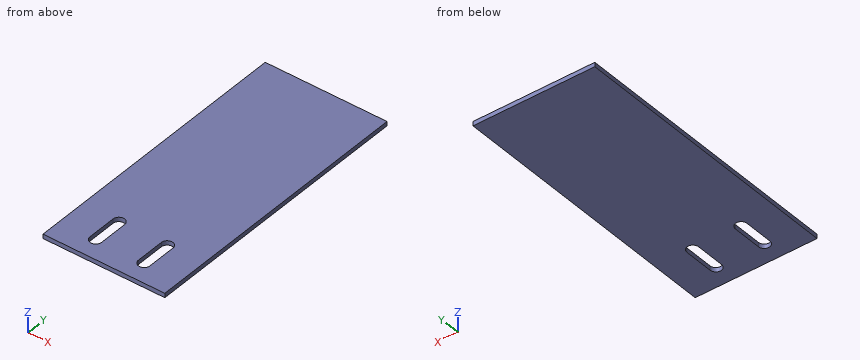
from build123d import *

# Parameters (mm, degrees)
SKETCH1_W           = 126
SKETCH1_H           = 290
BOSS_EXTRUDE2_DEPTH = 4.5


with BuildPart() as part:
    # Sketch1 → Boss-Extrude2 (new body)
    with BuildSketch(Plane.XY):
        Rectangle(SKETCH1_W, SKETCH1_H)
        with BuildLine():
            Line((-19, -109), (-19, -124))
            ThreePointArc((-19, -124), (-25, -130), (-31, -124))
            Line((-31, -124), (-31, -94))
            ThreePointArc((-31, -94), (-25, -88), (-19, -94))
            Line((-19, -94), (-19, -109))
        make_face(mode=Mode.SUBTRACT)
        with BuildLine():
            ThreePointArc((31, -124), (25, -130), (19, -124))
            Line((19, -124), (19, -94))
            ThreePointArc((19, -94), (25, -88), (31, -94))
            Line((31, -94), (31, -124))
        make_face(mode=Mode.SUBTRACT)
    extrude(amount=BOSS_EXTRUDE2_DEPTH)


solid = part.part
Input: part model. Units: mm. Frame: model coordinates. Coordinates: 2 decimals unless noted, no trailing zeros. Loops run counter-clockwise (first coordinate to the right, second up) from the corner with the lowest first, then second, coordinate; pieces in that order, holes last.
Q1. Cut plane B-B (z = 3.6). Output: boundary loops of the cut face in (x, y).
Q2. Cut plane C-C (x = -25). Output: boundary loops of the cut face in (y, z), then the cut area to 3 significant figures.
Q3. Cut plane A-A (y = -108). Output: boundary loops of the cut face in (x, z).
Q4. Material intervals for line 1 (X direction, y = -103, z = 3.05); line 2 (Y direction, x = -21, z = 3.5); line 3 (Y direction, x = 22.5, z = 0.95), sorted ascending.
Working result:
1. outline: (-63, -145) - (63, -145) - (63, 145) - (-63, 145) - close; hole (-31, -124) arc R6 ccw to (-19, -124) - (-19, -94) arc R6 ccw to (-31, -94) - close; hole (19, -124) arc R6 ccw to (31, -124) - (31, -94) arc R6 ccw to (19, -94) - close
2. outline: (-145, 0) - (-130, 0) - (-130, 4.5) - (-145, 4.5) - close; (-88, 0) - (145, 0) - (145, 4.5) - (-88, 4.5) - close
2. area: 1,120 mm2
3. outline: (-63, 0) - (-31, 0) - (-31, 4.5) - (-63, 4.5) - close; (-19, 0) - (19, 0) - (19, 4.5) - (-19, 4.5) - close; (31, 0) - (63, 0) - (63, 4.5) - (31, 4.5) - close
4. line 1: x = -63 to -31, -19 to 19, 31 to 63
4. line 2: y = -145 to -128.47, -89.53 to 145
4. line 3: y = -145 to -129.45, -88.55 to 145
